Could you check a few things on this model? Use its own coordinates, in mm. Give positions to 0.01 mm unless a question says otherwise; leave off trailing zeros. Order: outer loops, then holes, each group sorted by start corner. A loop starts at its lowest first (then second) coordinate and runs counter-clockwise, first axis right, second up.
(1) If I drill on probe 1 along Y at (x, z) = (0, 2.75); probe 2 along Y at (x, z) = (133.35, 4.75) (3 decimals); probe 3 along X at (y, z) = (61, 6), over which ranges is the centre line in solid material (lowest first)?
(2) Imagine slicing it at A-A, the plane x = 0. Write out the boundary of the cut face in (y, z) (3 decimals), then the cut area to 3 significant figures.
(3) Imagine slicing it at D-D, the plane z = 6.25. State how many separate pieces and enclosed holes the cut face has, then the cut area to 4 significant figures.
(4) Imagine slicing it at C-C, the plane x = -100.5. Write out the boundary of the cut face in (y, z) (3 decimals).
(5) Imagine slicing it at B-B, the plane y = -104. Write out the boundary of the cut face in (x, z) (3 decimals), then the cut area to 3 significant figures.
(6) Will these pins go through, and if not, where does the flat tip stop? pin 1 (4 mm diameter, centred on x = 198.44, y = -136.65, fed in from -Z); pin 2 (4 mm diameter, centred on x = -113.5, z = 2.5, fed in from +Y); pin 3 (1 mm diameter, centred on y = 132.5, z = 8, fed in from -X); pin 4 (1 mm diameter, centred on x = 75.5, z = 5, fed in from +Y).
from build123d import *

# Parameters (mm, degrees)
SKETCH1_R           = 127
SKETCH1_R_2         = 8.198770857
SKETCH1_R_3         = 6.35
SKETCH1_R_4         = 3.175
SKETCH1_R_5         = 9.525
BOSS_EXTRUDE1_DEPTH = 9.525


with BuildPart() as part:
    # Sketch1 → Boss-Extrude1 (new body)
    with BuildSketch(Plane.XY):
        with BuildLine():
            Line((-228.6, -36.83), (-228.6, -189.23))
            Line((-228.6, -189.23), (228.6, -189.23))
            Line((228.6, -189.23), (228.6, -36.83))
            ThreePointArc((228.6, -36.83), (0, 191.77), (-228.6, -36.83))
        make_face()
        with Locations(Location((0, 0, 0), (0, 0, 180))):
            Circle(SKETCH1_R, mode=Mode.SUBTRACT)
        with Locations(Location((0, 148.2852, 0), (0, 0, 180))):
            Circle(SKETCH1_R_2, mode=Mode.SUBTRACT)
        with Locations(Location((128.418750205, -74.1426, 0), (0, 0, 180))):
            Circle(SKETCH1_R_2, mode=Mode.SUBTRACT)
        with Locations(Location((-128.418750205, -74.1426, 0), (0, 0, 180))):
            Circle(SKETCH1_R_2, mode=Mode.SUBTRACT)
        with Locations(Location((203.2, -151.13, 0), (0, 0, 180))):
            Circle(SKETCH1_R_3, mode=Mode.SUBTRACT)
        with Locations(Location((188.723253344, -155.8925, 0), (0, 0, 180))):
            Circle(SKETCH1_R_4, mode=Mode.SUBTRACT)
        with Locations(Location((198.4375, -136.653253344, 0), (0, 0, 180))):
            Circle(SKETCH1_R_4, mode=Mode.SUBTRACT)
        with Locations(Location((133.35, -158.75, 0), (0, 0, 180))):
            Circle(SKETCH1_R_5, mode=Mode.SUBTRACT)
    extrude(amount=BOSS_EXTRUDE1_DEPTH)


solid = part.part
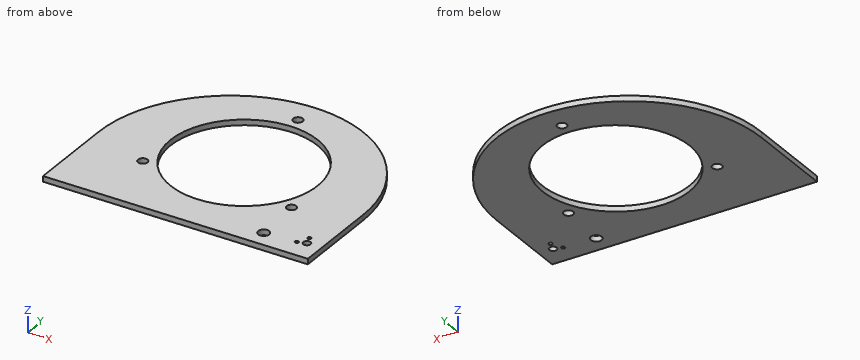
Answer block:
1. probe 1: y = -189.23 to -127, 127 to 140.09, 156.48 to 191.77
1. probe 2: y = -189.23 to -168.275, -149.225 to -80.693, -67.593 to 148.846
1. probe 3: x = -206.61 to -111.39, 111.39 to 206.61
2. outline: (-189.23, 0) - (-127, 0) - (-127, 9.525) - (-189.23, 9.525) - close; (127, 0) - (140.086, 0) - (140.086, 9.525) - (127, 9.525) - close; (156.484, 0) - (191.77, 0) - (191.77, 9.525) - (156.484, 9.525) - close
2. area: 1,050 mm2
3. separate pieces: 1
3. enclosed holes: 8
3. area: 100,000 mm2
4. outline: (-189.23, 0) - (-77.645, 0) - (-77.645, 9.525) - (-189.23, 9.525) - close; (77.645, 0) - (168.493, 0) - (168.493, 9.525) - (77.645, 9.525) - close
5. outline: (-228.6, 0) - (-72.89, 0) - (-72.89, 9.525) - (-228.6, 9.525) - close; (72.89, 0) - (228.6, 0) - (228.6, 9.525) - (72.89, 9.525) - close
5. area: 2,970 mm2
6. pin 1: passes through
6. pin 2: stops at y = 162.73
6. pin 3: stops at x = -154.12
6. pin 4: stops at y = 179.12
